Geometry check sheet. Reference: drawing and pictorial views, mm from the part's lowest x, y, z. A direction names the side the tool comes from. Coordinates: 2 decimals unless noted, no trailing zeros. Write each loop counter-clockwise with the first axis right and the second up, starting at its lowest first coordinate (ties: lowest second). Pieces come first, ordered by that corner, then holes. Notation, with made-up numbers: (13, -29.75) - (19, -29.75) arc R17 cw to (19, 2.25) - close; hole circle Ø7 at (61.25, 24.25). An arc over 180 degrees is marked (long way). Use one line per item in the form item = value. Start each with the question number.
(1) Gauge pin test, flat ends, axial feed: pin 1 Ø1 at (x, z) = (18, 13) entering from +Y; pin 2 Ø6 at (y, z) = (8, 14.5) entering from -X. Record the tip position at first contact, or that the pin passes through.
(2) Sectioned sample at D-D (x = 56). Record the cut outline in (y, z).
(3) Sectioned sample at B-B (x = 75). Record the cut outline in (y, z).
(4) Tool access check on the marked faces 1 and 2. Record the directions out of +Z, -Z, +X, -X, +Y, -Y that give a thin tool (end or side, any length) a straight path to the whole face; none if there is none.
(5) Sectioned sample at A-A (y = 24.5). Record the cut outline in (x, z), and give its area (3 significant figures).
(6) Sectioned sample at C-C (y = 45). Record the cut outline in (x, z).
(7) Material ranges on line 1 (Y direction, x = 75, z = 1); line 2 (Y direction, x = 46, z = 32), recorded low to high. Write a range as [from, to].
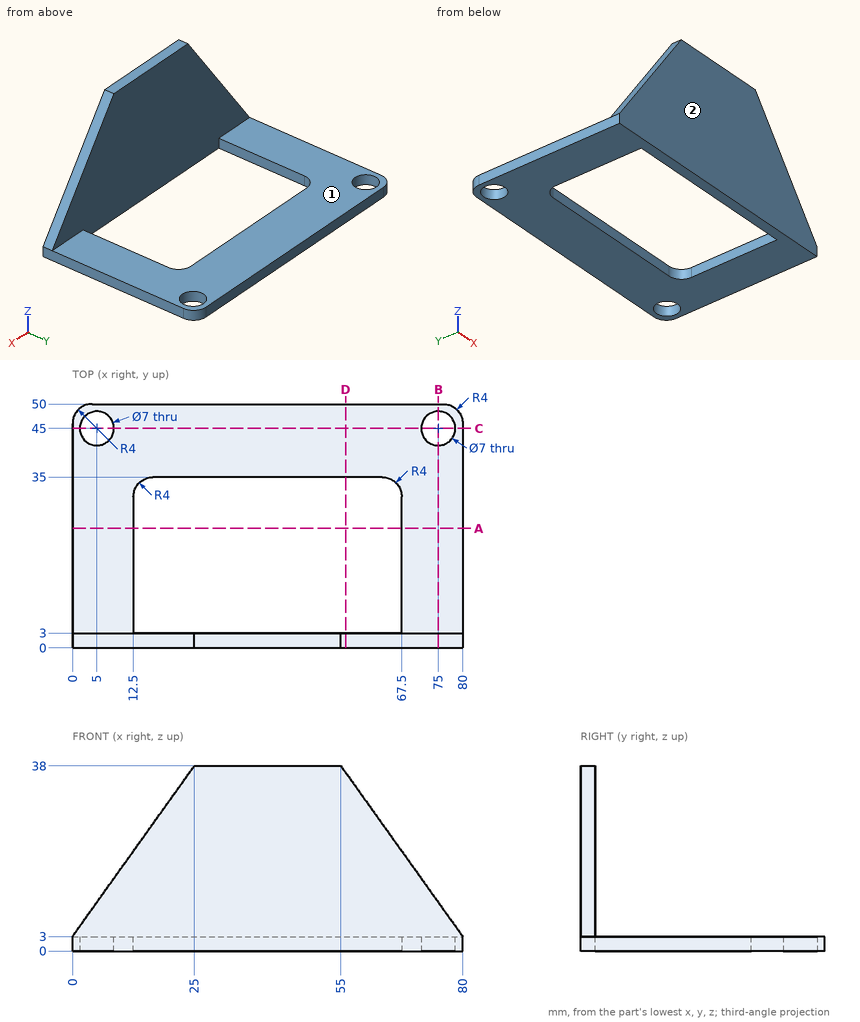
Answers below:
q1.pin_1 = 3
q1.pin_2 = through
q2.outline = (0, 0) - (3, 0) - (3, 36.6) - (0, 36.6) - close; (35, 0) - (50, 0) - (50, 3) - (35, 3) - close
q3.outline = (0, 0) - (41.5, 0) - (41.5, 3) - (3, 3) - (3, 10) - (0, 10) - close; (48.5, 0) - (50, 0) - (50, 3) - (48.5, 3) - close
q4.face_1 = +Z, +X, -X, +Y
q4.face_2 = +Z, -Z, +X, -X, -Y
q5.outline = (0, 0) - (12.5, 0) - (12.5, 3) - (0, 3) - close; (67.5, 0) - (80, 0) - (80, 3) - (67.5, 3) - close
q5.area = 75.0 mm2
q6.outline = (0, 0) - (1.5, 0) - (1.5, 3) - (0, 3) - close; (8.5, 0) - (71.5, 0) - (71.5, 3) - (8.5, 3) - close; (78.5, 0) - (80, 0) - (80, 3) - (78.5, 3) - close
q7.line_1 = [0, 41.5], [48.5, 50]
q7.line_2 = [0, 3]
